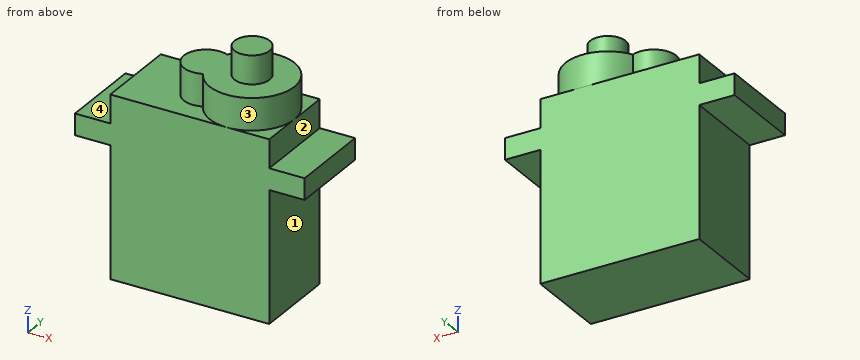
Autodesk Fusion 360 part; units mm, degrees
sketch "Sketch1" plane through (0, 0, 0) normal (0, 1, 0) x (1, 0, 0)
  line L0 (0, 0) -> (5, 0)
  line L1 (5, 0) -> (27.5, 0)
  line L2 (27.5, 0) -> (27.5, -18.5)
  line L3 (5, -18.5) -> (5, 0)
  line L4 (5, -21.5) -> (0, -21.5)
  line L5 (0, -21.5) -> (0, -18.5)
  line L6 (0, -18.5) -> (5, -18.5)
  line L7 (27.5, -21.5) -> (32.5, -21.5)
  line L8 (32.5, -21.5) -> (32.5, -18.5)
  line L9 (32.5, -18.5) -> (27.5, -18.5)
  line L10 (27.5, -21.5) -> (27.5, -25.5)
  line L11 (27.5, -25.5) -> (5, -25.5)
  line L12 (5, -25.5) -> (5, -21.5)
  dimension "d1" = 5
  dimension "d2" = 22.5
  dimension "d3" = 18.5
  dimension "d4" = 3
  dimension "d5" = 5
  dimension "d6" = 3
  dimension "d7" = 5
  dimension "d8" = 22.5
  dimension "d9" = 4
extrude "Extrude1" add sketch "Sketch1" along normal blind 12
sketch "Sketch2" plane through (0, 0, 25.5) normal (0, 0, 1) x (-1, 0, 0)
  line L0 (-5, 0) -> (-27.5, 0)
  line L1 (-27.5, 0) -> (-27.5, -12)
  line L2 (-27.5, -12) -> (-5, -12)
  line L3 (-5, -12) -> (-5, 0)
  circle A0 centre (-21.5, -6) radius 6
  circle A1 centre (-15, -6) radius 3.15
  dimension "d14" = 6.3
extrude "Extrude2" add sketch "Sketch2" along normal blind 4.5 contours A0 A1 | A0 A1 picked at (-24.363, -5.7154) picked at (-16.388, -6.4033)
extrude "Extrude3" add sketch "Sketch2" along normal blind 4.5 contours A0 A1 picked at (-14.3919, -6.6826)
sketch "Sketch3" plane through (0, 0, 30) normal (0, 0, 1) x (-1, 0, 0)
  arc A0 (-16.244, -3.1061) -> (-16.244, -8.8939) centre (-21.5, -6) ccw
  arc A1 (-16.244, -8.8939) -> (-16.244, -3.1061) centre (-15, -6) ccw
  circle A2 centre (-21.5, -6) radius 2.5
  dimension "d17" = 5
extrude "Extrude4" add sketch "Sketch3" along normal blind 4 contours A2
Could you check a few things on this model? Use its own coordinates, in mm. Face numbers are marked on the shaded views. A direction names the side the tool comes from. Give positions to 0.01 mm unless a question says otherwise; leave off trailing zeros. Loops run counter-clockwise (first coordinate to the right, second up) from the corner with the lowest first, then second, coordinate; pieces in that order, holes last. Notation, with made-up numbers: M -7,50 L 27,50 A14 cw 27,60 Z; hole C 24,52.25 d4. An arc over 180 degrees is marked long. Answer as a JSON object with one key per item and string values.
Q1. If I drill on probe 1 along X at (y, z) = (10.5, 15); probe 2 along Z at (x, y) = (4.5, 0.5); probe 3 along Z at (x, y) = (27, 2.25), over which ranges is the centre line in solid material (lowest first)? Write a range as [from, to].
Values found:
{"probe 1": "x = [5, 27.5]", "probe 2": "z = [18.5, 21.5]", "probe 3": "z = [0, 25.5]"}
Q2. Suppose I cut it at C-C, the plane y = 1.5. List the corners of the cut face in (x, z) for me.
Values found:
{"outline": "M 0,18.5 L 5,18.5 L 5,0 L 27.5,0 L 27.5,18.5 L 32.5,18.5 L 32.5,21.5 L 27.5,21.5 L 27.5,25.5 L 25.47,25.5 L 25.47,30 L 17.53,30 L 17.53,25.5 L 5,25.5 L 5,21.5 L 0,21.5 Z"}
Q3. For P1, Ø2, axis at y = 4, z = 23, coming from the +X side; P2, Ø3.5, axis at y = 9, z = 12, coming from the -X side; P3, Ø5.5, axis at x = 2.5, y = 7, coming from the +Z side, each with a flat end and sliding along its axis, tell me the tip position at first contact or that it passes through.
Values found:
{"P1": "stops at x = 27.5", "P2": "stops at x = 5", "P3": "stops at z = 25.5"}
Q4. Suppose I cut it at B-B, the plane z = 17. List the corners of the cut face in (x, y) for me, plus the area to 3 significant figures.
Values found:
{"outline": "M 5,0 L 27.5,0 L 27.5,12 L 5,12 Z", "area": "270 mm²"}
Q5. Suppose I cut it at A-A, the plane x = 15. List the corners of the cut face in (y, z) for me, plus the area to 3 significant figures.
Values found:
{"outline": "M 0,0 L 12,0 L 12,25.5 L 9.15,25.5 L 9.15,30 L 2.85,30 L 2.85,25.5 L 0,25.5 Z", "area": "334 mm²"}
Q6. Suppose I cut it at D-D, the plane x = 7.5. List the corners of the cut face in (y, z) for me.
Values found:
{"outline": "M 0,0 L 12,0 L 12,25.5 L 0,25.5 Z"}
Q7. For the marked faces 1, 2, 3 and 4, which set-ups out of +Z, -Z, +X, -X, +Y, -Y let a thin tool reach every point of the face, with its end or its side?
Values found:
{"face 1": "-Z, +X, +Y, -Y", "face 2": "+Z, +X, +Y, -Y", "face 3": "+Z", "face 4": "+Z, -X, +Y, -Y"}
